Check sheet for the modelled part. Datum: model origin and axes. Units: mm. A direction names the side the tool comes from. Give positions to 0.01 mm unless a question says otherwise; leave off trailing zeros. Write each loop counter-clockwise with the first axis right and the second up, starting at its lowest first coordinate (ties: lowest second). Pieces come first, ordered by that corner, then holes. Notation, with made-up numbers: M 79.25,-8.75 L 105.25,-8.75 A4 ccw 105.25,-1.75 Z; hole C -13,23.25 d7. An arc over 180 degrees is marked long. Use CSV: the item, a comma, the result in double quotes. Start each with the question number.
1. Mould release check, pull along X, two halves, no side actions. Record for faces 5 (the face through (43, 20, 5)), 6 (the face through (45.5, 25, 4.9)): +X half, -X half, draft (parallel to the pull), parting line (faces both ways), or undercut.
2. Scan line: line 1 (Y direction, x = 34, z = 2.5). Record every from-to range of solid material in increasing order.
3. Access from +Z, -Z, +X, -X, +Y, -Y to the whole of each face (thin tool, end or side, straight path). Record for faces 1 (the face through (38, 20, 5)), 2 (the face through (41, 2, 5)), 3 (the face through (16, 12, 5)), 4 (the face through (10.5, 25, 4.9)).
4. Depth check by flat-ended pin: P1, Ø1.2, axis at x = 28.5, z = 7, coming from the -Y side; P2, Ø3, axis at x = 28, z = 7.5, coming from the +Y side; P3, Ø1.2, axis at y = 6.5, z = 3, coming from the -X side. Enter the tip coordinate at first touch or a pass-through.
5. Cross-section at A-A, the plane x = 37. Enter the section's corners in (y, z), and give its area (3 significant figures).
6. Cross-section at B-B, the plane y = 12.5. State how many separate pieces and enclosed holes the cut face has, and give its area (3 significant figures).
from build123d import *

# Parameters (mm, degrees)
F0_W     = 4
F0_H     = 4
F1_DEPTH = 10


with BuildPart() as f1:
    # F0 (on Top) → F1 (new body)
    with BuildSketch(Plane.XY):
        Polygon((0, 5), (0, 4), (1, 4), (5, 4), (5, 0), (6, 0), (6, 4), (10, 4), (10, 0), (11, 0), (11, 4), (15, 4), (15, 0), (16, 0), (16, 4), (20, 4), (20, 0), (21, 0), (21, 4), (25, 4), (25, 0), (26, 0), (26, 4), (30, 4), (30, 0), (31, 0), (31, 4), (35, 4), (35, 0), (36, 0), (36, 4), (40, 4), (40, 0), (41, 0), (41, 4), (45, 4), (45, 0), (46, 0), (46, 4), (50, 4), (50, 5), (46, 5), (46, 9), (50, 9), (50, 10), (46, 10), (46, 14), (50, 14), (50, 15), (46, 15), (46, 19), (50, 19), (50, 20), (46, 20), (46, 24), (46, 25), (45, 25), (45, 24), (45, 20), (41, 20), (41, 24), (41, 25), (40, 25), (40, 24), (40, 20), (36, 20), (36, 24), (36, 25), (35, 25), (35, 24), (35, 20), (31, 20), (31, 24), (31, 25), (30, 25), (30, 24), (30, 20), (26, 20), (26, 24), (26, 25), (25, 25), (25, 24), (25, 20), (21, 20), (21, 24), (21, 25), (20, 25), (20, 24), (20, 20), (16, 20), (16, 24), (16, 25), (15, 25), (15, 24), (15, 20), (11, 20), (11, 24), (11, 25), (10, 25), (10, 24), (10, 20), (6, 20), (6, 24), (6, 25), (5, 25), (5, 24), (5, 20), (1, 20), (0, 20), (0, 19), (1, 19), (5, 19), (5, 15), (1, 15), (0, 15), (0, 14), (1, 14), (5, 14), (5, 10), (1, 10), (0, 10), (0, 9), (1, 9), (5, 9), (5, 5), (1, 5), align=None)
        with Locations((8, 7)):
            Rectangle(F0_W, F0_H, mode=Mode.SUBTRACT)
        with Locations((8, 12)):
            Rectangle(F0_W, F0_H, mode=Mode.SUBTRACT)
        with Locations((13, 7)):
            Rectangle(F0_W, F0_H, mode=Mode.SUBTRACT)
        with Locations((18, 7)):
            Rectangle(F0_W, F0_H, mode=Mode.SUBTRACT)
        with Locations((23, 7)):
            Rectangle(F0_W, F0_H, mode=Mode.SUBTRACT)
        with Locations((13, 12)):
            Rectangle(F0_W, F0_H, mode=Mode.SUBTRACT)
        with Locations((18, 12)):
            Rectangle(F0_W, F0_H, mode=Mode.SUBTRACT)
        with Locations((23, 12)):
            Rectangle(F0_W, F0_H, mode=Mode.SUBTRACT)
        with Locations((28, 7)):
            Rectangle(F0_W, F0_H, mode=Mode.SUBTRACT)
        with Locations((33, 7)):
            Rectangle(F0_W, F0_H, mode=Mode.SUBTRACT)
        with Locations((28, 12)):
            Rectangle(F0_W, F0_H, mode=Mode.SUBTRACT)
        with Locations((33, 12)):
            Rectangle(F0_W, F0_H, mode=Mode.SUBTRACT)
        with Locations((38, 7)):
            Rectangle(F0_W, F0_H, mode=Mode.SUBTRACT)
        with Locations((43, 7)):
            Rectangle(F0_W, F0_H, mode=Mode.SUBTRACT)
        with Locations((38, 12)):
            Rectangle(F0_W, F0_H, mode=Mode.SUBTRACT)
        with Locations((43, 12)):
            Rectangle(F0_W, F0_H, mode=Mode.SUBTRACT)
        with Locations((8, 17)):
            Rectangle(F0_W, F0_H, mode=Mode.SUBTRACT)
        with Locations((13, 17)):
            Rectangle(F0_W, F0_H, mode=Mode.SUBTRACT)
        with Locations((18, 17)):
            Rectangle(F0_W, F0_H, mode=Mode.SUBTRACT)
        with Locations((23, 17)):
            Rectangle(F0_W, F0_H, mode=Mode.SUBTRACT)
        with Locations((28, 17)):
            Rectangle(F0_W, F0_H, mode=Mode.SUBTRACT)
        with Locations((33, 17)):
            Rectangle(F0_W, F0_H, mode=Mode.SUBTRACT)
        with Locations((38, 17)):
            Rectangle(F0_W, F0_H, mode=Mode.SUBTRACT)
        with Locations((43, 17)):
            Rectangle(F0_W, F0_H, mode=Mode.SUBTRACT)
    extrude(amount=F1_DEPTH)


solid = f1.part
Worked answers:
1,face 5,"undercut"
1,face 6,"draft"
2,line 1,"y = 4 to 5, 9 to 10, 14 to 15, 19 to 20"
3,face 1,"+Z, -Z, +Y"
3,face 2,"+Z, -Z, -Y"
3,face 3,"+Z, -Z"
3,face 4,"+Z, -Z, +X, -X, +Y"
4,P1,"stops at y = 4"
4,P2,"stops at y = 20"
4,P3,"stops at x = 5"
5,outline,"M 4,0 L 5,0 L 5,10 L 4,10 Z; M 9,0 L 10,0 L 10,10 L 9,10 Z; M 14,0 L 15,0 L 15,10 L 14,10 Z; M 19,0 L 20,0 L 20,10 L 19,10 Z"
5,area,"40.0 mm^2"
6,separate pieces,"9"
6,enclosed holes,"0"
6,area,"90.0 mm^2"
